```python
from build123d import *

# Parameters (mm, degrees)
SKETCH_1_R      = 1.6
SKETCH_1_R_2    = 17.5
SKETCH_1_W      = 2
SKETCH_1_H      = 15
EXTRUDE_1_DEPTH = 3
FILLET_2_R      = 4


with BuildPart() as part:
    # 草图1 → 凸台-拉伸1 (new body)
    with BuildSketch(Plane(origin=(0, 0, 0), x_dir=(1, 0, 0), z_dir=(0, 1, 0))):
        with BuildLine():
            Line((-65, 65), (65, 65))
            Line((65, 65), (65, 55))
            ThreePointArc((65, 55), (67.928932188, 47.928932188), (75, 45))
            Line((75, 45), (100, 45))
            Line((100, 45), (100, -45))
            Line((100, -45), (75, -45))
            ThreePointArc((75, -45), (67.928932188, -47.928932188), (65, -55))
            Line((65, -55), (65, -65))
            Line((65, -65), (-65, -65))
            Line((-65, -65), (-65, -55))
            ThreePointArc((-65, -55), (-67.928932188, -47.928932188), (-75, -45))
            Line((-75, -45), (-100, -45))
            Line((-100, -45), (-100, 45))
            Line((-100, 45), (-75, 45))
            ThreePointArc((-75, 45), (-67.928932188, 47.928932188), (-65, 55))
            Line((-65, 55), (-65, 65))
        make_face()
        with Locations(Location((-47.93, 47.93, 0), (0, 0, 270))):
            Circle(SKETCH_1_R, mode=Mode.SUBTRACT)
        with Locations(Location((49.344213562, 49.344213562, 0), (0, 0, 270))):
            Circle(SKETCH_1_R, mode=Mode.SUBTRACT)
        with Locations(Location((50.758427125, -47.93, 0), (0, 0, 270))):
            Circle(SKETCH_1_R, mode=Mode.SUBTRACT)
        with Locations(Location((-46.515786438, -49.344213562, 0), (0, 0, 270))):
            Circle(SKETCH_1_R, mode=Mode.SUBTRACT)
        with Locations(Location((43, -29, 0), (0, 0, 270))):
            Circle(SKETCH_1_R, mode=Mode.SUBTRACT)
        with Locations(Location((-43, -29, 0), (0, 0, 270))):
            Circle(SKETCH_1_R, mode=Mode.SUBTRACT)
        with Locations(Location((-43, 29, 0), (0, 0, 270))):
            Circle(SKETCH_1_R, mode=Mode.SUBTRACT)
        with Locations(Location((43, 29, 0), (0, 0, 270))):
            Circle(SKETCH_1_R, mode=Mode.SUBTRACT)
        with Locations(Location((0, 0, 0), (0, 0, 270))):
            Circle(SKETCH_1_R_2, mode=Mode.SUBTRACT)
        with Locations(Location((-95.757359313, 40.757359313, 0), (0, 0, 270))):
            Circle(SKETCH_1_R, mode=Mode.SUBTRACT)
        with Locations(Location((95.757359313, 40.757359313, 0), (0, 0, 270))):
            Circle(SKETCH_1_R, mode=Mode.SUBTRACT)
        with Locations(Location((95.757359313, -40.757359313, 0), (0, 0, 270))):
            Circle(SKETCH_1_R, mode=Mode.SUBTRACT)
        with Locations(Location((-95.757359313, -40.757359313, 0), (0, 0, 270))):
            Circle(SKETCH_1_R, mode=Mode.SUBTRACT)
        with Locations((-84.2325, 0)):
            Rectangle(SKETCH_1_W, SKETCH_1_H, mode=Mode.SUBTRACT)
        with BuildLine():
            Line((-48.465, 10), (-48.465, -10))
            ThreePointArc((-48.465, -10), (-56.465, -18), (-64.465, -10))
            Line((-64.465, -10), (-64.465, 10))
            ThreePointArc((-64.465, 10), (-56.465, 18), (-48.465, 10))
        make_face(mode=Mode.SUBTRACT)
        with BuildLine():
            Line((48.465, 10), (48.465, -10))
            ThreePointArc((48.465, -10), (56.465, -18), (64.465, -10))
            Line((64.465, -10), (64.465, 10))
            ThreePointArc((64.465, 10), (56.465, 18), (48.465, 10))
        make_face(mode=Mode.SUBTRACT)
        with BuildLine():
            Line((-25, 52.93), (25, 52.93))
            ThreePointArc((25, 52.93), (30, 47.93), (25, 42.93))
            Line((25, 42.93), (-25, 42.93))
            ThreePointArc((-25, 42.93), (-30, 47.93), (-25, 52.93))
        make_face(mode=Mode.SUBTRACT)
        with BuildLine():
            Line((-25, -52.93), (25, -52.93))
            ThreePointArc((25, -52.93), (30, -47.93), (25, -42.93))
            Line((25, -42.93), (-25, -42.93))
            ThreePointArc((-25, -42.93), (-30, -47.93), (-25, -52.93))
        make_face(mode=Mode.SUBTRACT)
        with Locations((-72.2325, 0)):
            Rectangle(SKETCH_1_W, SKETCH_1_H, mode=Mode.SUBTRACT)
        with Locations((-84.2325, -25)):
            Rectangle(SKETCH_1_W, SKETCH_1_H, mode=Mode.SUBTRACT)
        with Locations((-72.2325, -25)):
            Rectangle(SKETCH_1_W, SKETCH_1_H, mode=Mode.SUBTRACT)
        with Locations((-72.2325, 25)):
            Rectangle(SKETCH_1_W, SKETCH_1_H, mode=Mode.SUBTRACT)
        with Locations((-84.2325, 25)):
            Rectangle(SKETCH_1_W, SKETCH_1_H, mode=Mode.SUBTRACT)
        with Locations((84.2325, 25)):
            Rectangle(SKETCH_1_W, SKETCH_1_H, mode=Mode.SUBTRACT)
        with Locations((72.2325, 25)):
            Rectangle(SKETCH_1_W, SKETCH_1_H, mode=Mode.SUBTRACT)
        with Locations((84.2325, 0)):
            Rectangle(SKETCH_1_W, SKETCH_1_H, mode=Mode.SUBTRACT)
        with Locations((72.2325, 0)):
            Rectangle(SKETCH_1_W, SKETCH_1_H, mode=Mode.SUBTRACT)
        with Locations((84.2325, -25)):
            Rectangle(SKETCH_1_W, SKETCH_1_H, mode=Mode.SUBTRACT)
        with Locations((72.2325, -25)):
            Rectangle(SKETCH_1_W, SKETCH_1_H, mode=Mode.SUBTRACT)
    extrude(amount=EXTRUDE_1_DEPTH)

    # 圆角2
    fillet_2_edges = [part.edges().sort_by_distance(p)[0] for p in [
        (100, 1.5, -45),
        (100, 1.5, 45),
        (65, 1.5, 65),
        (-65, 1.5, 65),
        (-100, 1.5, 45),
        (-100, 1.5, -45),
        (-65, 1.5, -65),
        (65, 1.5, -65),
    ]]
    fillet(fillet_2_edges, radius=FILLET_2_R)


solid = part.part
```
Model file for the job. Use its own axes, mm. A direction names the side the tool comes from. Coordinates: 2 decimals unless noted, no trailing zeros. Write each loop counter-clockwise with the first axis right and the second up, starting at its lowest first coordinate (ties: lowest second). Pieces come first, ordered by that corner, then holes. Notation, with made-up numbers: (-7.5, 59) - (23.5, 59) arc R26 cw to (23.5, 74) - close; hole circle Ø11 at (80.25, -11). An arc over 180 degrees is marked (long way). One line per item, written item: value. Start each with the question number.
1. Mould opens along Z. For faces 1 (the cylindrical face through (-98.797, 1.521, -43.859)), 2 (the cylindrical face through (-30, 1, 48)), 3 (the cylindrical face through (63.859, 1.521, 63.797)) say: released by +Z, released by -Z, zero draft, split by the parting line, or undercut.
2. Slice it at A-A (z = -23). Write the cut outline in (x, y).
3. Tool access for faces 4 (the cylindrical face through (98.797, 1.521, -43.859)), 5 (the cylindrical face through (-56.3, 1.5, 18)): list every direction of +Z, -Z, +X, -X, +Y, -Y with a clear straight run to the whole face (end or side of a thin tool).
4. Probe line 1 (X direction, y = 1.45, z = 20); line 2 (Z direction, x = 21, y = 2.7); line 3 (Z direction, x = 5, y = 0.85). List the from-to ranges inside material, lowest first. Write a range as from..to.
5. Slice it at C-C (y = 1.05). Count the separate pieces of the cut face and the enclosed holes in it, plus the area to 3 significant figures.
6. Flat gauge pins, fed straight in: pin 1 (4 mm diameter, centred on x = -43, z = 29, fed in from -Y); pin 2 (1 mm diameter, centred on x = 84, y = 1, fed in from +Z); pin 3 (0.6 mm diameter, centred on x = 72, y = 1, fed in from -Z); pin 4 (0.6 mm diameter, centred on x = -72.5, y = 1, fed in from +Z). Where does each tip first touch, or does it go through?
7. Slice it at B-B (x = -21). Write the cut outline in (y, z), plus the area to 3 significant figures.
Answers below:
1. face 1: released by -Z
1. face 2: undercut
1. face 3: released by +Z
2. outline: (-100, 0) - (-85.23, 0) - (-85.23, 3) - (-100, 3) - close; (-83.23, 0) - (-73.23, 0) - (-73.23, 3) - (-83.23, 3) - close; (-71.23, 0) - (71.23, 0) - (71.23, 3) - (-71.23, 3) - close; (73.23, 0) - (83.23, 0) - (83.23, 3) - (73.23, 3) - close; (85.23, 0) - (100, 0) - (100, 3) - (85.23, 3) - close
3. face 4: -Z, +X, +Y, -Y
3. face 5: +Y, -Y
4. line 1: x = -100..-85.23, -83.23..-73.23, -71.23..71.23, 73.23..83.23, 85.23..100
4. line 2: z = -65..-52.93, -42.93..42.93, 52.93..65
4. line 3: z = -65..-52.93, -42.93..-16.77, 16.77..42.93, 52.93..65
5. separate pieces: 1
5. enclosed holes: 29
5. area: 19,600 mm^2
6. pin 1: stops at y = 0
6. pin 2: stops at z = 45
6. pin 3: stops at z = -45.56
6. pin 4: stops at z = 45.4
7. outline: (0, -65) - (3, -65) - (3, -52.93) - (0, -52.93) - close; (0, -42.93) - (3, -42.93) - (3, 42.93) - (0, 42.93) - close; (0, 52.93) - (3, 52.93) - (3, 65) - (0, 65) - close
7. area: 330 mm^2
